Build history of the part. All positions in model axes, mm. Face numbers are marked on the shaded views. A direction names the side the tool comes from. Round coordinates to 2 decimals unless told otherwise and drop trailing zeros. Write each loop counter-clockwise with the first axis right and the second up, starting at its lowest first coordinate (ties: lowest second). Pieces come first, ordered by that corner, then holes.
Item 1: 3-axis set-ups, long thin cutter, end or side, ignore diameter. For the marked faces 5 and 6: which of +Z, -Z, +X, -X, +Y, -Y reach the whole face in a straight line?
Item 2: Mould opens along Z. For the marked faces 1, 2, 3 and 4 say: +Z half, -Z half, draft (parallel to the pull), parting line (faces both ways), or undercut.
Item 3: Band-saw the part on B-B, the plane y = 1.85. Write the cut outline in (x, z), then the cut area to 3 significant figures.
Item 4: Wall check: probe 1 along X at (y, z) = (4.2, 0); probe 2 along X at (y, z) = (1.9, 0); probe 3 along Y at (x, z) = (-6, -1.5). Give the ranges that are in metal, low to high.
Item 5: Band-saw the part on A-A, the plane z = 0. Write the cut outline in (x, y), then the cut area to 3 significant figures.
```python
from build123d import *

# Parameters (mm, degrees)
SKETCH_4_R          = 11.6
SKETCH_4_R_2        = 1.1
EXTRUDE_1_DEPTH     = 1.1
EXTRUDE_START       = 1.5
SKETCH_4_3_R        = 9
SKETCH_4_3_R_2      = 1.1
EXTRUDE_2_DEPTH     = 3.3
CHAMFER_1_SIZE      = 0.2
SKETCH_6_R          = 7.35
SKETCH_6_R_2        = 4.5
CUT_EXTRUDE_1_DEPTH = 1
CHAMFER_2_SIZE      = 0.4
SKETCH_4_4_R        = 1.1
CUT_EXTRUDE_2_DEPTH = 18.092688495
CHAMFER_3_SIZE      = 0.5


with BuildPart() as part:
    # Sketch 4 → Extrude 1 (new body)
    with BuildSketch(Plane(origin=(0, 0, 0), x_dir=(1, 0, 0), z_dir=(0, 1, 0))):
        with Locations(Location((0, 0, 0), (0, 0, 270))):
            Circle(SKETCH_4_R)
        with Locations(Location((0, 0, 0), (0, 0, 270))):
            Circle(SKETCH_4_R_2, mode=Mode.SUBTRACT)
    extrude(amount=EXTRUDE_1_DEPTH)

    # Chamfer 1
    chamfer_1_edges = [part.edges().sort_by_distance(p)[0] for p in [
        (0, 1.1, -11.6),
    ]]
    chamfer(chamfer_1_edges, length=CHAMFER_1_SIZE)


with BuildPart() as body_2:
    # Sketch 4_3 → Extrude 2 (new body)
    with BuildSketch(Plane(origin=(0, 0, 0), x_dir=(1, 0, 0), z_dir=(0, 1, 0)).offset(EXTRUDE_START)):
        with Locations(Location((0, 0, 0), (0, 0, 270))):
            Circle(SKETCH_4_3_R)
        with Locations(Location((0, 0, 0), (0, 0, 270))):
            Circle(SKETCH_4_3_R_2, mode=Mode.SUBTRACT)
    extrude(amount=EXTRUDE_2_DEPTH)


    add(part.part)  # loft_1 joins it to this body
    # loft up to a face of the part (loft_1)
    loft([Face(Wire([body_2.edges().sort_by_distance((-6.560717647, 1.5, -6.160923953))[0]])), Face(Wire([body_2.edges().sort_by_distance((8.310242353, 1.1, -7.803837008))[0]]))])

    # Sketch 6 → Cut-Extrude 1 (cut)
    with BuildSketch(Plane(origin=(0, 4.8, 0), x_dir=(1, 0, 0), z_dir=(0, 1, 0))):
        with Locations(Location((0, 0, 0), (0, 0, 270))):
            Circle(SKETCH_6_R)
        with Locations(Location((0, 0, 0), (0, 0, 270))):
            Circle(SKETCH_6_R_2, mode=Mode.SUBTRACT)
    extrude(amount=-CUT_EXTRUDE_1_DEPTH, mode=Mode.SUBTRACT)

    # Chamfer 2
    chamfer_2_edges = [body_2.edges().sort_by_distance(p)[0] for p in [
        (0, 4.8, -9),
        (0, 4.8, -4.5),
    ]]
    chamfer(chamfer_2_edges, length=CHAMFER_2_SIZE)

    # Sketch 4_4 → Cut-Extrude 2 (cut, through all)
    with BuildSketch(Plane(origin=(0, 0, 0), x_dir=(1, 0, 0), z_dir=(0, 1, 0))):
        with Locations(Location((0, 0, 0), (0, 0, 270))):
            Circle(SKETCH_4_4_R)
    extrude(amount=CUT_EXTRUDE_2_DEPTH, mode=Mode.SUBTRACT)

    # Chamfer 3
    chamfer_3_edges = [body_2.edges().sort_by_distance(p)[0] for p in [
        (0, 0, -1.1),
    ]]
    chamfer(chamfer_3_edges, length=CHAMFER_3_SIZE)


solid = body_2.part
```
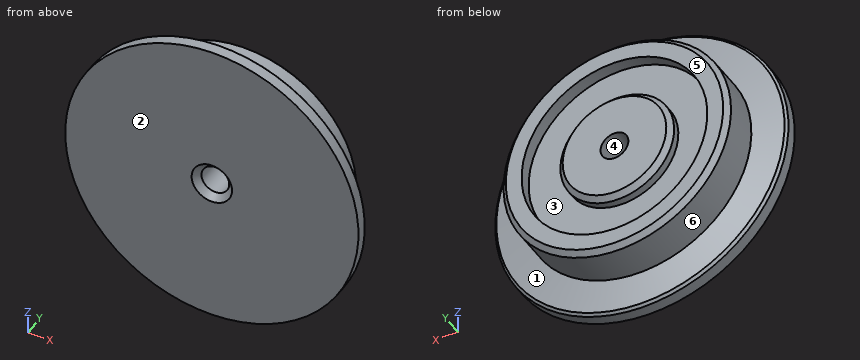
Results:
1. face 5: +Z, -Z, +X, -X, +Y
1. face 6: +Y
2. face 1: parting line
2. face 2: draft
2. face 3: undercut
2. face 4: undercut
3. outline: circle Ø18 at (0, 0); hole circle Ø2.2 at (0, 0)
3. area: 251 mm2
4. probe 1: x = -9 to -7.35, -4.5 to -1.1, 1.1 to 4.5, 7.35 to 9
4. probe 2: x = -9 to -1.1, 1.1 to 9
4. probe 3: y = 0 to 3.8
5. outline: (-11.6, 0) - (-1.6, 0) - (-1.1, 0.5) - (-1.1, 4.8) - (-4.1, 4.8) - (-4.5, 4.4) - (-4.5, 3.8) - (-7.35, 3.8) - (-7.35, 4.8) - (-8.6, 4.8) - (-9, 4.4) - (-9, 1.5) - (-11.4, 1.1) - (-11.6, 0.9) - close; (1.1, 0.5) - (1.6, 0) - (11.6, 0) - (11.6, 0.9) - (11.4, 1.1) - (9, 1.5) - (9, 4.4) - (8.6, 4.8) - (7.35, 4.8) - (7.35, 3.8) - (4.5, 3.8) - (4.5, 4.4) - (4.1, 4.8) - (1.1, 4.8) - close
5. area: 76.2 mm2
